Can you work these out from the model? Positions are in its coordinate system, mm. Round coordinates to 2 decimals unless told otherwise and drop trailing zeros. Write each loop counter-clockwise with the first axis right and the second up, starting at its lowest first coordinate (ties: lowest second). Pieces come first, ordered by that corner, then holes. Notation, with made-up numbers: M 65.25,-0.5 L 118.25,-0.5 A10 ccw 118.25,14.5 Z; hole C -5.75,53.5 d7. An arc over 180 degrees is marked long. Answer as a JSON object with one key per item and string values. Group by question number.
1) Suppose I cut it at C-C, the plane z = 0.5. Write out the boundary of the cut face in (x, y), and give its area (3 significant figures).
2) Suppose I cut it at B-B, the plane x = 63. Write out the boundary of the cut face in (y, z).
3) Please list where these lines run through material, in increasing order: L1, parallel to X at y = 4.25, z = -68; L2, parallel to Z at x = 82, y = 0.45; L3, parallel to Z at x = -26.5, y = 2.1. Write a range as [from, to].
4) Suppose I cut it at A-A, the plane y = 1.5. State how many separate pieces and enclosed holes the cut face has, and give its area (3 significant figures).
5) I'm going to push flat-ended pins straight in: pin 1 Ø1 at (y, z) = (0.5, -43) entering from -X; pin 2 Ø3 at (x, y) = (85.5, 1.5) entering from +Z; pin 3 Ø2 at (y, z) = (1.5, -72) entering from -X; pin 4 Ø1 at (x, z) = (-28, 5) entering from -Y. Where does each tip first touch, or does it pass through?
from build123d import *

# Parameters (mm, degrees)
RESSALTO_EXTRUS_O2_DEPTH = 5
CORTE_EXTRUS_O1_DEPTH    = 5


with BuildPart() as part:
    # Esboço1 → Ressalto-extrusão2 (new body)
    with BuildSketch(Plane(origin=(0, 0, 0), x_dir=(1, 0, 0), z_dir=(0, 1, 0))):
        with BuildLine():
            Line((-50.542684331, 81.382727595), (-18.443667531, 113.481744396))
            ThreePointArc((-18.443667531, 113.481744396), (-16.222396505, 114.770390532), (-13.65444113, 114.786484772))
            ThreePointArc((-13.65444113, 114.786484772), (38.248428139, 108.173840066), (90.151297409, 114.786484772))
            ThreePointArc((90.151297409, 114.786484772), (92.719252784, 114.770390532), (94.94052381, 113.481744396))
            Line((94.94052381, 113.481744396), (127.03954061, 81.382727595))
            ThreePointArc((127.03954061, 81.382727595), (127.79593841, 80.412212643), (128.29241049, 79.286356356))
            ThreePointArc((128.29241049, 79.286356356), (136.248428139, 25.173840066), (128.29241049, -28.938676225))
            ThreePointArc((128.29241049, -28.938676225), (127.79593841, -30.064532511), (127.03954061, -31.035047464))
            Line((127.03954061, -31.035047464), (94.94052381, -63.134064264))
            ThreePointArc((94.94052381, -63.134064264), (92.719252784, -64.4227104), (90.151297409, -64.438804641))
            ThreePointArc((90.151297409, -64.438804641), (38.248428139, -57.826159934), (-13.65444113, -64.438804641))
            ThreePointArc((-13.65444113, -64.438804641), (-16.222396505, -64.4227104), (-18.443667531, -63.134064264))
            Line((-18.443667531, -63.134064264), (-50.542684331, -31.035047464))
            ThreePointArc((-50.542684331, -31.035047464), (-51.299082131, -30.064532511), (-51.795554211, -28.938676225))
            ThreePointArc((-51.795554211, -28.938676225), (-59.751571861, 25.173840066), (-51.795554211, 79.286356356))
            ThreePointArc((-51.795554211, 79.286356356), (-51.299082131, 80.412212643), (-50.542684331, 81.382727595))
        make_face()
    extrude(amount=RESSALTO_EXTRUS_O2_DEPTH)

    # Esboço2 → Corte-extrusão1 (cut)
    with BuildSketch(Plane(origin=(0, 5, 0), x_dir=(1, 0, 0), z_dir=(0, 1, 0))):
        with BuildLine():
            Line((-30.957642025, 93.896702089), (-45.049304874, 79.805039241))
            ThreePointArc((-45.049304874, 79.805039241), (-46.07443114, 77.330165506), (-45.049304874, 74.855291772))
            Line((-45.049304874, 74.855291772), (-35.856916719, 65.662903617))
            ThreePointArc((-35.856916719, 65.662903617), (-33.382042984, 64.637777351), (-30.90716925, 65.662903617))
            Line((-30.90716925, 65.662903617), (-1.915791222, 94.654281645))
            ThreePointArc((-1.915791222, 94.654281645), (-0.890664956, 97.12915538), (-1.915791222, 99.604029114))
            Line((-1.915791222, 99.604029114), (-11.108179377, 108.796417269))
            ThreePointArc((-11.108179377, 108.796417269), (-13.583053111, 109.821543535), (-16.057926845, 108.796417269))
            Line((-16.057926845, 108.796417269), (-30.957642025, 93.896702089))
        make_face()
        with BuildLine():
            Line((-30.957642025, -43.549021958), (-16.057926845, -58.448737138))
            ThreePointArc((-16.057926845, -58.448737138), (-13.583053111, -59.473863403), (-11.108179377, -58.448737138))
            Line((-11.108179377, -58.448737138), (-1.915791222, -49.256348982))
            ThreePointArc((-1.915791222, -49.256348982), (-0.890664956, -46.781475248), (-1.915791222, -44.306601514))
            Line((-1.915791222, -44.306601514), (-30.90716925, -15.315223485))
            ThreePointArc((-30.90716925, -15.315223485), (-33.382042984, -14.290097219), (-35.856916719, -15.315223485))
            Line((-35.856916719, -15.315223485), (-45.049304874, -24.507611641))
            ThreePointArc((-45.049304874, -24.507611641), (-46.07443114, -26.982485375), (-45.049304874, -29.457359109))
            Line((-45.049304874, -29.457359109), (-30.957642025, -43.549021958))
        make_face()
        with BuildLine():
            Line((107.454498304, -43.549021958), (121.546161153, -29.457359109))
            ThreePointArc((121.546161153, -29.457359109), (122.571287419, -26.982485375), (121.546161153, -24.507611641))
            Line((121.546161153, -24.507611641), (112.353772997, -15.315223485))
            ThreePointArc((112.353772997, -15.315223485), (109.878899263, -14.290097219), (107.404025529, -15.315223485))
            Line((107.404025529, -15.315223485), (78.4126475, -44.306601514))
            ThreePointArc((78.4126475, -44.306601514), (77.387521235, -46.781475248), (78.4126475, -49.256348982))
            Line((78.4126475, -49.256348982), (87.605035656, -58.448737138))
            ThreePointArc((87.605035656, -58.448737138), (90.07990939, -59.473863403), (92.554783124, -58.448737138))
            Line((92.554783124, -58.448737138), (107.454498304, -43.549021958))
        make_face()
        with BuildLine():
            Line((87.605035656, 108.796417269), (78.4126475, 99.604029114))
            ThreePointArc((78.4126475, 99.604029114), (77.387521235, 97.12915538), (78.4126475, 94.654281645))
            Line((78.4126475, 94.654281645), (107.404025529, 65.662903617))
            ThreePointArc((107.404025529, 65.662903617), (109.878899263, 64.637777351), (112.353772997, 65.662903617))
            Line((112.353772997, 65.662903617), (121.546161153, 74.855291772))
            ThreePointArc((121.546161153, 74.855291772), (122.571287419, 77.330165506), (121.546161153, 79.805039241))
            Line((121.546161153, 79.805039241), (107.454498304, 93.896702089))
            Line((107.454498304, 93.896702089), (92.554783124, 108.796417269))
            ThreePointArc((92.554783124, 108.796417269), (90.07990939, 109.821543535), (87.605035656, 108.796417269))
        make_face()
    extrude(amount=-CORTE_EXTRUS_O1_DEPTH, mode=Mode.SUBTRACT)


solid = part.part
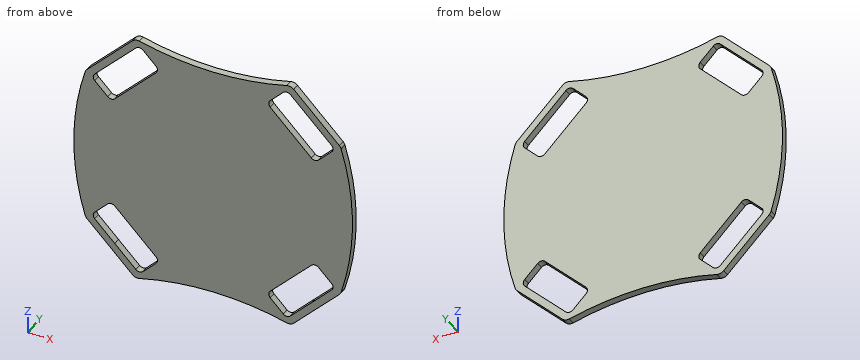
Results:
{
 "1": {"outline": "M -57.99,0 L 134.49,0 L 134.49,5 L -57.99,5 Z", "area": "962 mm^2"},
 "2": {"outline": "M 0,-109.66 L 5,-109.66 L 5,59.31 L 0,59.31 Z"},
 "3": {"L1": "[-54.81, -38.19], [-28.57, 105.07], [114.69, 131.31]", "L2": "[-112.85, -103.19], [-91.07, 40.72], [52.84, 62.5]", "L3": "[-105.43, -98.35], [-70.07, 19.72], [48.01, 55.08]"},
 "4": {"separate pieces": "1", "enclosed holes": "4", "area": "26,300 mm^2"},
 "5": {"pin 1": "x = -58.95", "pin 2": "z = 63.65", "pin 3": "x = -54.08", "pin 4": "y = 0"}
}
